Job drawing, mm, ordinate dimensions from the low corner. One solid piece. A direction names the side the tool comes from. Give positions to 0.01 mm unless a question says otherwise; leave off trailing zeros. Loops run counter-clockwise (first coordinate to the right, second up) from the corner with the lowest first, then second, coordinate; pieces in that order, holes last. Notation, with made-up numbers: (12, 39.25) -> (68, 39.25) arc R17 cw to (68, 65.25) -> close; hole circle Ø4 at (52.25, -37). An arc over 180 degrees is marked (long way). Use one line per item in the form item = value.
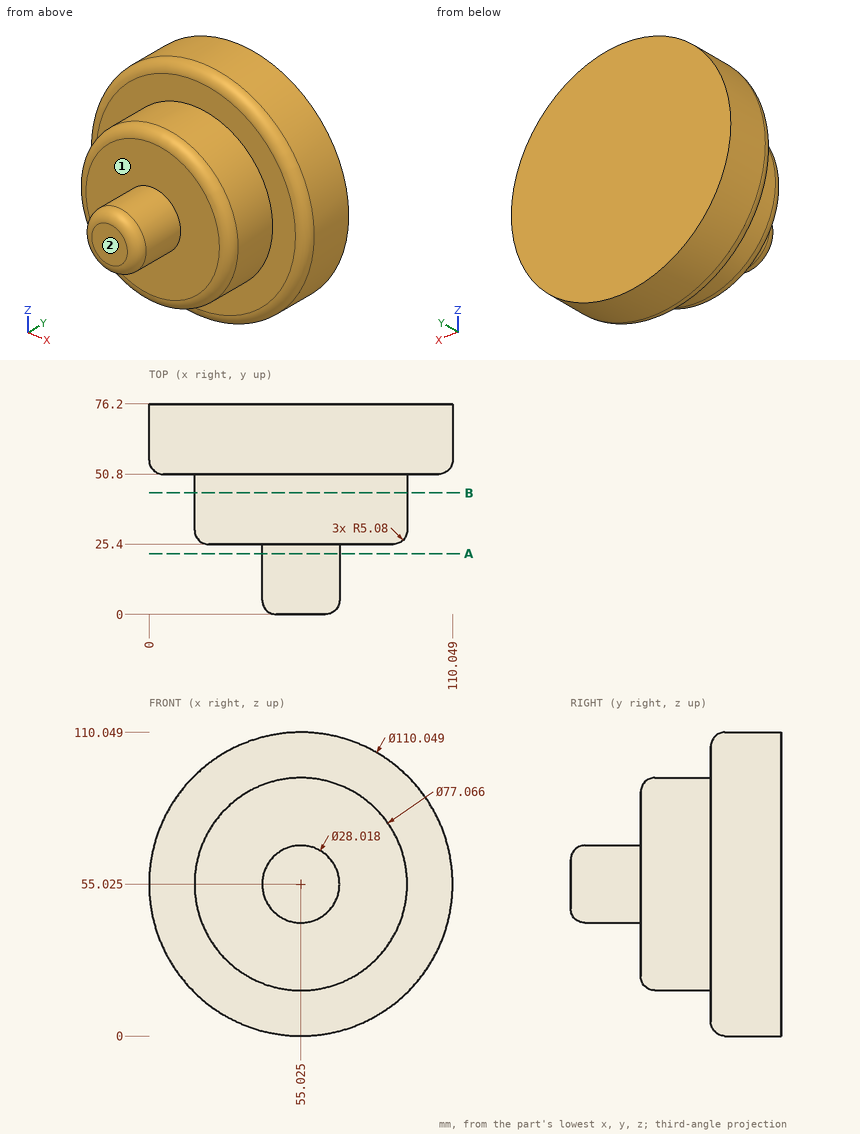
1. Cut at B-B, the plane y = 44. Write the cut outline in (x, z) (1 decimal).
Result sheet:
outline = circle Ø77.1 at (55, 55)
2. Tool access for the marked faces 1 and 2: list every direction of +Z, -Z, +X, -X, +Y, -Y with a clear straight run to the whole face (end or side of a thin tool).
Result sheet:
face_1 = -Y
face_2 = +Z, -Z, +X, -X, -Y
3. Drop flat-ended pins along their axis: P1, Ø8, axis at y = 61.5, z = 81, coming from the -X side; P2, Ø2, axis at x = 63.5, y = 67.5, coming from the -Z side; P3, Ø4, axis at y = 29.5, z = 56.5, coming from the +X side. Give the stop position or say it passes through.
Result sheet:
P1 = 4.58
P2 = 0.51
P3 = 93.56
4. Cut at A-A, the plane y = 22. Write the cut outline in (x, z) (1 decimal).
Result sheet:
outline = circle Ø28 at (55, 55)
5. Drill centre lines: line 1 (Y direction, x = 77.5, z = 39); line 2 (Y direction, x = 102, z = 43); line 3 (X direction, y = 37, z = 57). Where is each one in solid material? Low to high.
Result sheet:
line_1 = 25.4 to 76.2
line_2 = 50.8 to 76.2
line_3 = 16.54 to 93.51
